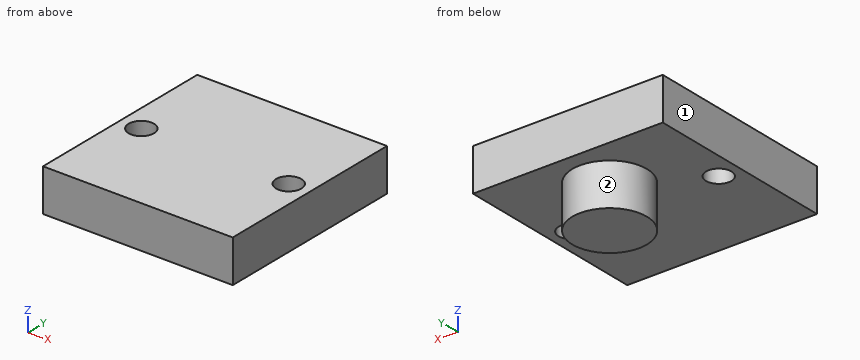
from build123d import *

# Parameters (mm, degrees)
SKETCH1_W           = 22.4
SKETCH1_H           = 22.9
BOSS_EXTRUDE1_DEPTH = 5
SKETCH2_R           = 1.5
CUT_EXTRUDE1_DEPTH  = 5
SKETCH4_R           = 4.4
BOSS_EXTRUDE3_DEPTH = 5


with BuildPart() as part:
    # Sketch1 → Boss-Extrude1 (new body)
    with BuildSketch(Plane.XY):
        Rectangle(SKETCH1_W, SKETCH1_H)
    extrude(amount=BOSS_EXTRUDE1_DEPTH)

    # Sketch2 → Cut-Extrude1 (cut)
    with BuildSketch(Plane.XY.offset(5)):
        with Locations((-8.7, 0)):
            Circle(SKETCH2_R)
        with Locations((8.7, 0)):
            Circle(SKETCH2_R)
    extrude(amount=-CUT_EXTRUDE1_DEPTH, mode=Mode.SUBTRACT)

    # Sketch4 → Boss-Extrude3 (add)
    with BuildSketch(Plane(origin=(0, 0, 0), x_dir=(-1, 0, 0), z_dir=(0, 0, -1))):
        with Locations((0, 5.25)):
            Circle(SKETCH4_R)
    extrude(amount=BOSS_EXTRUDE3_DEPTH)


solid = part.part
Verification items for the finished model (mm, model axes). Face numbers are marked on the shaded views. A direction names the side the tool comes from. Coordinates: 2 decimals unless noted, no trailing zeros. Write each loop counter-clockwise with the first axis right and the second up, starting at its lowest first coordinate (ties: lowest second). Pieces come first, ordered by that corner, then holes. Notation, with made-up numbers: (24, 41.5) -> (44, 41.5) arc R13 ccw to (44, 64.5) -> close; hole circle Ø1 at (10.5, 64.25). An arc over 180 degrees is marked (long way). One line per item, written item: value. Start each with the question number.
Q1. Cross-section at A-A on x = -8.7. Enter the section's corners in (y, z), and give its area (3 significant figures).
Q2. Access from +Z, -Z, +X, -X, +Y, -Y to the whole of each face (thin tool, end or side, straight path). Record for the marked faces 1 and 2.
Q3. Go/stop test with flat-tipped pins: P1, Ø3, axis at x = -7.5, y = -3.5, coming from the -Z side; P2, Ø1.5, axis at x = 1.5, z = -2.5, coming from the +Y side. Record where each tip stops, or that it passes through.
Q4. Cross-section at D-D on x = 0. Enter the section's corners in (y, z), and give its area (4 significant figures).
Q5. Cross-section at B-B on y = 5.25. Enter the section's corners in (x, z), and give its area (3 significant figures).
Q6. Thickness scan on L1, parallel to Y at x = -8.7, z = 3.4; L2, parallel to Z at x = 6, y = -9; L3, parallel to Y at x = 2.5, z = -4.5. Record the ranges inside material, lowest first. Write a range as from..to.
Q7. Cross-section at C-C on z = 2. Enter the section's corners in (x, y).
Checked values:
1. outline: (-11.45, 0) -> (-1.5, 0) -> (-1.5, 5) -> (-11.45, 5) -> close; (1.5, 0) -> (11.45, 0) -> (11.45, 5) -> (1.5, 5) -> close
1. area: 99.5 mm²
2. face 1: +Z, -Z, -X, +Y, -Y
2. face 2: -Z
3. P1: stops at z = 0
3. P2: stops at y = 9.59
4. outline: (-11.45, 0) -> (0.85, 0) -> (0.85, -5) -> (9.65, -5) -> (9.65, 0) -> (11.45, 0) -> (11.45, 5) -> (-11.45, 5) -> close
4. area: 158.5 mm²
5. outline: (-11.2, 0) -> (-4.4, 0) -> (-4.4, -5) -> (4.4, -5) -> (4.4, 0) -> (11.2, 0) -> (11.2, 5) -> (-11.2, 5) -> close
5. area: 156 mm²
6. L1: y = -11.45..-1.5, 1.5..11.45
6. L2: z = 0..5
6. L3: y = 1.63..8.87
7. outline: (-11.2, -11.45) -> (11.2, -11.45) -> (11.2, 11.45) -> (-11.2, 11.45) -> close; hole circle Ø3 at (-8.7, 0); hole circle Ø3 at (8.7, 0)
